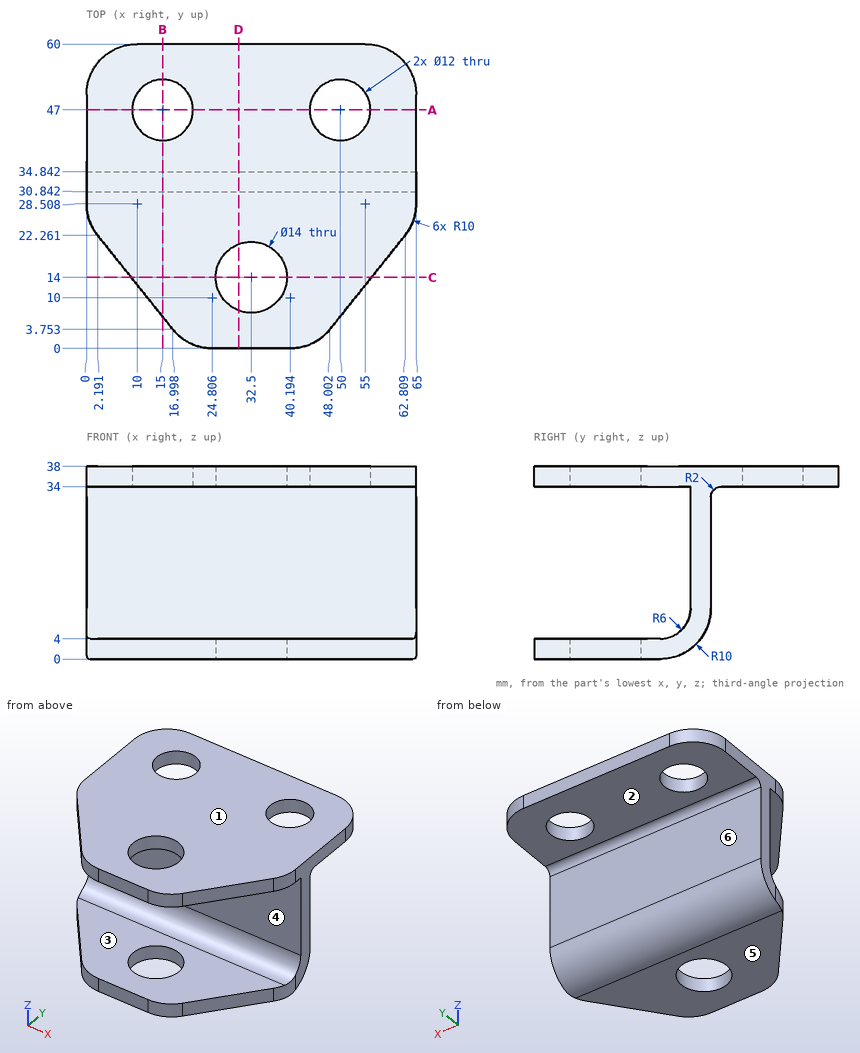
The drawing under review shows one solid part. Ordinate dimensions are in mm from its lowest x, y, z. A direction names the side the tool comes from. Give positions to 0.01 mm unless a question says otherwise; leave off trailing zeros. Loops run counter-clockwise (first coordinate to the right, second up) from the corner with the lowest first, then second, coordinate; pieces in that order, holes last. Notation, with made-up numbers: M 69,-30.5 L 111,-30.5 A19 ccw 111,4.5 Z; hole C -33,62.25 d10. An arc over 180 degrees is marked long. One line per question, with ' | ' between items. Start each with the question number.
1. Add section C-C (y = 14). Write out the cut boundary in (x, z), plus the area to 3 significant figures.
2. Insertion check: P1, Ø4, axis at x = 36.5, z = 10.5, coming from the +Y side; P2, Ø10, axis at y = 47, z = 32.5, coming from the +X side. Each pin has a flat end and moves straight along its axis. Give the tip position at first contact, or say it passes through.
3. The part is to be moulded in two halves that separate along Z. For the marked faces 1, 2 and 3, say which applies: released by +Z, released by -Z, zero draft, split by the parting line, or undercut.
4. To check wall thickness, follow L1, parallel to Y at x = 32, z = 36; L2, parallel to Z at x = 19, y = 10; L3, parallel to Y at x = 10, z = 14.5. State the ranges of each line that lie inside material, in increasing order.
5. For the marked faces 4, 5 and 6, list the 3-axis set-ups (+Z, -Z, +X, -X, +Y, -Y) from which the entire face can be reached by the end or side of a thin tool; tool diameter is ignored.
6. Add section A-A (y = 47). Write out the cut boundary in (x, z), plus the area to 3 significant figures.
7. Add section B-B (x = 15). Write out the cut boundary in (y, z).
8. Add section D-D (x = 30). Write out the cut boundary in (y, z).
Worked out:
1) outline: M 8.8,0 L 25.5,0 L 25.5,4 L 8.8,4 Z; M 8.8,34 L 25.5,34 L 25.5,38 L 8.8,38 Z; M 39.5,0 L 56.2,0 L 56.2,4 L 39.5,4 Z; M 39.5,34 L 56.2,34 L 56.2,38 L 39.5,38 Z | area: 267 mm²
2) P1: stops at y = 34.84 | P2: stops at x = 65
3) face 1: released by +Z | face 2: released by -Z | face 3: undercut
4) L1: y = 0 to 7.02, 20.98 to 60 | L2: z = 0 to 4, 34 to 38 | L3: y = 30.84 to 34.84
5) face 4: +X, -X, -Y | face 5: -Z, +X, -X, +Y, -Y | face 6: -Z, +X, -X, +Y
6) outline: M 0,34 L 9,34 L 9,38 L 0,38 Z; M 21,34 L 44,34 L 44,38 L 21,38 Z; M 56,34 L 65,34 L 65,38 L 56,38 Z | area: 164 mm²
7) outline: M 6.25,0 L 24.84,0 A10 ccw 34.84,10 L 34.84,32 A2 cw 36.84,34 L 41,34 L 41,38 L 6.25,38 L 6.25,34 L 30.84,34 L 30.84,10 A6 cw 24.84,4 L 6.25,4 Z; M 53,34 L 60,34 L 60,38 L 53,38 Z
8) outline: M 0,0 L 7.46,0 L 7.46,4 L 0,4 Z; M 0,34 L 7.46,34 L 7.46,38 L 0,38 Z; M 20.54,0 L 24.84,0 A10 ccw 34.84,10 L 34.84,32 A2 cw 36.84,34 L 60,34 L 60,38 L 20.54,38 L 20.54,34 L 30.84,34 L 30.84,10 A6 cw 24.84,4 L 20.54,4 Z
